from build123d import *

# Parameters (mm, degrees)
F0_W     = 89
F0_H     = 62
F0_R     = 2
F1_DEPTH = 3
F2_R     = 2.4
F3_DEPTH = 1.7


with BuildPart() as f1:
    # F0 (on Top) → F1 (new body)
    with BuildSketch(Plane.XY):
        Rectangle(F0_W, F0_H)
        with Locations((-40.5, -27)):
            Circle(F0_R, mode=Mode.SUBTRACT)
        with Locations((40.5, -27)):
            Circle(F0_R, mode=Mode.SUBTRACT)
        with Locations((-40.5, 27)):
            Circle(F0_R, mode=Mode.SUBTRACT)
        with Locations((40.5, 27)):
            Circle(F0_R, mode=Mode.SUBTRACT)
    extrude(amount=F1_DEPTH)

    # F2 (on face) → F3 (join)
    with BuildSketch(Plane.XY.offset(3)):
        with Locations((16, 21.304145)):
            Circle(F2_R)
        with Locations((24, 21.304145)):
            Circle(F2_R)
        with Locations((0, -10.695855)):
            Circle(F2_R)
        with Locations((8, -18.695855)):
            Circle(F2_R)
        with Locations((24, -18.695855)):
            Circle(F2_R)
        with Locations((0, -2.695855)):
            Circle(F2_R)
        with Locations((-8, -10.695855)):
            Circle(F2_R)
        with Locations((-24, 13.304145)):
            Circle(F2_R)
        with Locations((32, -18.695855)):
            Circle(F2_R)
        with Locations((-24, -18.695855)):
            Circle(F2_R)
        with Locations((8, 13.304145)):
            Circle(F2_R)
        with Locations((32, 21.304145)):
            Circle(F2_R)
        with Locations((16, -10.695855)):
            Circle(F2_R)
        with Locations((16, -18.695855)):
            Circle(F2_R)
        with Locations((24, -10.695855)):
            Circle(F2_R)
        with Locations((-8, -18.695855)):
            Circle(F2_R)
        with Locations((32, 13.304145)):
            Circle(F2_R)
        with Locations((-32, 21.304145)):
            Circle(F2_R)
        with Locations((-16, -18.695855)):
            Circle(F2_R)
        with Locations((0, 21.304145)):
            Circle(F2_R)
        with Locations((-16, 21.304145)):
            Circle(F2_R)
        with Locations((-16, -10.695855)):
            Circle(F2_R)
        with Locations((-8, 21.304145)):
            Circle(F2_R)
        with Locations((-32, -10.695855)):
            Circle(F2_R)
        with Locations((8, 21.304145)):
            Circle(F2_R)
        with Locations((-32, -18.695855)):
            Circle(F2_R)
        with Locations((-8, 13.304145)):
            Circle(F2_R)
        with Locations((-24, 21.304145)):
            Circle(F2_R)
        with Locations((-24, -10.695855)):
            Circle(F2_R)
        with Locations((32, -10.695855)):
            Circle(F2_R)
        with Locations((0, -18.695855)):
            Circle(F2_R)
        with Locations((8, -10.695855)):
            Circle(F2_R)
        with Locations((-16, -2.695855)):
            Circle(F2_R)
        with Locations((-24, -2.695855)):
            Circle(F2_R)
        with Locations((16, -2.695855)):
            Circle(F2_R)
        with Locations((24, -2.695855)):
            Circle(F2_R)
        with Locations((-32, -2.695855)):
            Circle(F2_R)
        with Locations((8, -2.695855)):
            Circle(F2_R)
        with Locations((32, -2.695855)):
            Circle(F2_R)
        with Locations((-8, -2.695855)):
            Circle(F2_R)
        with Locations((0, 5.304145)):
            Circle(F2_R)
        with Locations((-16, 5.304145)):
            Circle(F2_R)
        with Locations((-24, 5.304145)):
            Circle(F2_R)
        with Locations((16, 5.304145)):
            Circle(F2_R)
        with Locations((24, 5.304145)):
            Circle(F2_R)
        with Locations((-32, 5.304145)):
            Circle(F2_R)
        with Locations((8, 5.304145)):
            Circle(F2_R)
        with Locations((32, 5.304145)):
            Circle(F2_R)
        with Locations((16, 13.304145)):
            Circle(F2_R)
        with Locations((-8, 5.304145)):
            Circle(F2_R)
        with Locations((0, 13.304145)):
            Circle(F2_R)
        with Locations((-16, 13.304145)):
            Circle(F2_R)
        with Locations((24, 13.304145)):
            Circle(F2_R)
        with Locations((-32, 13.304145)):
            Circle(F2_R)
    extrude(amount=F3_DEPTH)


solid = f1.part
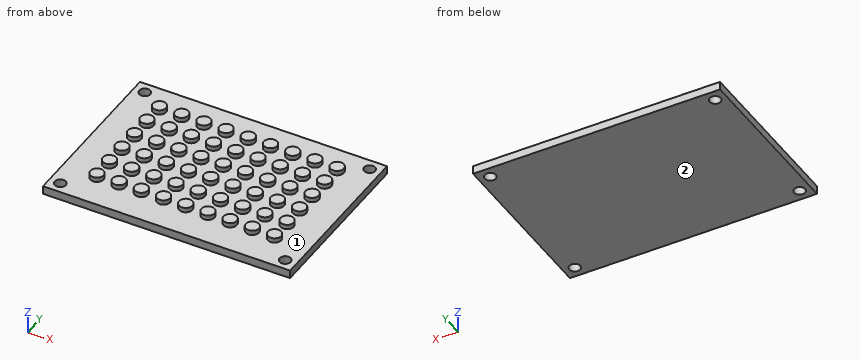
Could you check a few things on this model? Use its own coordinates, in mm. Face numbers are marked on the shaded views. Give positions to 0.01 mm unless a question says otherwise; leave off trailing zeros. Order: outer loops, then holes, each group sorted by start corner. A loop starts at its lowest first (then second) coordinate and runs counter-clockwise, first axis right, second up.
Item 1: If we section it at B-B, the plane x = 40.5: Write out the boundary of the cut face in (y, z), plus the area to 3 significant figures.
Item 2: I need wall thicknesses on line 1 (Y direction, x = -40.5, z = 0.9); line 2 (Y direction, x = 24.5, z = 4.05); line 3 (Y direction, x = 9.5, z = 3.3). Which ranges of each line are inside material? Lowest first, please.
Item 3: If we section it at C-C, the plane x = -8: Write out the boundary of the cut face in (y, z), plus the area to 3 significant figures.
Item 4: If we section it at A-A, the plane y = -27: Write out the boundary of the cut face in (x, z).
Item 5: If we mould it in two halves opening along Y, with no side actions, what happens to the marked faces 1 and 2? For each: pulls with the +Y half, pulls with the -Y half, needs draft (parallel to the pull), parting line crosses it, or undercut.
Item 6: I'm going to push flat-ended pins straight in: pin 1 (6.5 mm diameter, centred on x = 40.5, y = 27, fed in from +Z); pin 2 (6.5 mm diameter, centred on x = -40.5, y = -27, fed in from -Z); pin 3 (2.5 mm diameter, centred on x = -40.5, y = 27, fed in from -Z). Where does each tip first touch, or does it pass through?
Item 7: If we section it at D-D, the plane z = 3.8: Count the separate pieces of the cut face and the enclosed holes in it, plus the area to 3 significant figures.
Values:
1. outline: (-31, 0) - (-29, 0) - (-29, 3) - (-31, 3) - close; (-25, 0) - (25, 0) - (25, 3) - (-25, 3) - close; (29, 0) - (31, 0) - (31, 3) - (29, 3) - close
1. area: 162 mm2
2. line 1: y = -31 to -29, -25 to 25, 29 to 31
2. line 2: y = -21.04 to -16.35, -13.04 to -8.35, -5.04 to -0.35, 2.96 to 7.65, 10.96 to 15.65, 18.96 to 23.65
2. line 3: y = -20.57 to -16.82, -12.57 to -8.82, -4.57 to -0.82, 3.43 to 7.18, 11.43 to 15.18, 19.43 to 23.18
3. outline: (-31, 0) - (31, 0) - (31, 3) - (23.7, 3) - (23.7, 4.7) - (18.9, 4.7) - (18.9, 3) - (15.7, 3) - (15.7, 4.7) - (10.9, 4.7) - (10.9, 3) - (7.7, 3) - (7.7, 4.7) - (2.9, 4.7) - (2.9, 3) - (-0.3, 3) - (-0.3, 4.7) - (-5.1, 4.7) - (-5.1, 3) - (-8.3, 3) - (-8.3, 4.7) - (-13.1, 4.7) - (-13.1, 3) - (-16.3, 3) - (-16.3, 4.7) - (-21.1, 4.7) - (-21.1, 3) - (-31, 3) - close
3. area: 235 mm2
4. outline: (-44.5, 0) - (-42.5, 0) - (-42.5, 3) - (-44.5, 3) - close; (-38.5, 0) - (38.5, 0) - (38.5, 3) - (-38.5, 3) - close; (42.5, 0) - (44.5, 0) - (44.5, 3) - (42.5, 3) - close
5. face 1: undercut
5. face 2: needs draft
6. pin 1: stops at z = 3
6. pin 2: stops at z = 0
6. pin 3: passes through
7. separate pieces: 54
7. enclosed holes: 0
7. area: 977 mm2
